Geometry check sheet. Reference: the model listing, model coordinates, mm. Face numbers are marked on the shaded views. A direction names the side the tool comes from. Round coordinates to 2 decimals unless told otherwise and drop trailing zeros. Write each loop counter-clockwise with the first axis right and the second up, starting at its lowest first coordinate (ties: lowest second). Pieces come first, ordered by that corner, then holes.
Item 1: Draft check along X on the marked faces 6, 7 and 8. Enter one of: pulls with the +X half, pulls with the -X half, needs draft (parallel to the pull), parting line crosses it, or undercut.
Item 2: Cross-section at C-C (x = 102.5). Enter the section's corners in (y, z) (3 decimals).
Item 3: Cross-section at B-B (y = 37). Enter the section's corners in (x, z) (3 decimals).
Item 4: Scan lines: probe 1 along Z at (x, y) = (21, 10) (3 decimals); probe 2 along Z at (x, y) = (69, -11) (3 decimals); probe 3 along Y at (x, z) = (11, 49). Record each from-to range of solid material in increasing order.
Item 5: Cross-section at A-A (z = -2.5). Enter the section's corners in (x, y) (3 decimals).
Item 6: Access from +Z, -Z, +X, -X, +Y, -Y to the whole of each face (thin tool, end or side, straight path). Record for the marked faces 1, 2, 3, 4 and 5.
Item 7: Depth check by flat-ended pin: P1, Ø11, axis at y = -7.5, z = 12.5, coming from the +X side (3 decimals); P2, Ø5, axis at y = -15.5, z = 20, coming from the -X side (3 decimals); P3, Ø15.5, axis at x = 20, z = 27, coming from the +Y side; P4, Ø12, axis at x = 36.5, z = 8, coming from the -Y side. Enter the tip coordinate at first touch or a pass-through.
from build123d import *

# Parameters (mm, degrees)
F1_DEPTH = 63.5
F2_DEPTH = 25.4
F0_W     = 25.4
F0_H     = 19.05
F3_DEPTH = 25.4
F4_DEPTH = 7.9375
F6_R     = 6.35


with BuildPart() as f1:
    # F0 (on Front) → F1 (new body, symmetric)
    with BuildSketch(Plane.XZ):
        Polygon((22.225, 9.525), (-41.275, 9.525), (-41.275, -9.525), (41.275, -9.525), (41.275, 9.525), align=None)
    extrude(amount=F1_DEPTH, both=True)

    # F0 (on Front) → F2 (join, symmetric)
    with BuildSketch(Plane.XZ):
        with BuildLine():
            Line((22.225, 27.0002), (22.225, 9.525))
            Line((22.225, 9.525), (41.275, 9.525))
            Line((41.275, 9.525), (41.275, 27.0002))
            ThreePointArc((41.275, 27.0002), (45.9246798487, 38.2255201513), (57.15, 42.8752))
            Line((57.15, 42.8752), (60.325, 42.8752))
            Line((60.325, 42.8752), (60.325, 61.9252))
            Line((60.325, 61.9252), (57.15, 61.9252))
            add(Edge.make_bspline(
                [(56.5114887891, 61.9193627682), (56.7252668459, 61.9225827874), (56.9381101801, 61.9245325067), (57.15, 61.9252)],
                knots=[110.8414409639, 110.8414409639, 110.8414409639, 110.8414409639, 111.5045361635, 111.5045361635, 111.5045361635, 111.5045361635], degree=3))
            ThreePointArc((56.5114887891, 61.9193627682), (32.2295703384, 51.469115188), (22.225, 27.0002))
        make_face()
    extrude(amount=F2_DEPTH, both=True)

    # F0 (on Front) → F3 (join, symmetric)
    with BuildSketch(Plane.XZ):
        with Locations((73.025, 52.4002)):
            Rectangle(F0_W, F0_H)
    extrude(amount=F3_DEPTH, both=True)

    # F0 (on Front) → F4 (join, symmetric)
    with BuildSketch(Plane.XZ):
        with BuildLine():
            add(Edge.make_bspline(
                [(-41.275, 9.525), (-41.0755103707, 25.3485469245), (20.7768493641, 61.3811119099), (56.5114887891, 61.9193627682)],
                knots=[0, 0, 0, 0, 110.8414409639, 110.8414409639, 110.8414409639, 110.8414409639], degree=3))
            Line((-41.275, 9.525), (22.225, 9.525))
            Line((22.225, 9.525), (22.225, 27.0002))
            ThreePointArc((22.225, 27.0002), (32.2295703384, 51.469115188), (56.5114887891, 61.9193627682))
        make_face()
    extrude(amount=F4_DEPTH, both=True)

    # F0 (on Front) → F5 (revolve)
    with BuildSketch(Plane.XZ):
        Polygon((85.725, 66.675), (85.725, 61.9252), (85.725, 42.8752), (85.725, 38.1), (111.125, 38.1), (111.125, 66.675), align=None)
    revolve(axis=Axis((85.725, 0, 52.3875), (0, 0, 1)))

    # F6
    f6_edges = [f1.edges().sort_by_distance(p)[0] for p in [
        (-41.275, -63.5, 0),
        (41.275, -63.5, 0),
        (41.275, 63.5, 0),
        (-41.275, 63.5, 0),
    ]]
    fillet(f6_edges, radius=F6_R)


solid = f1.part
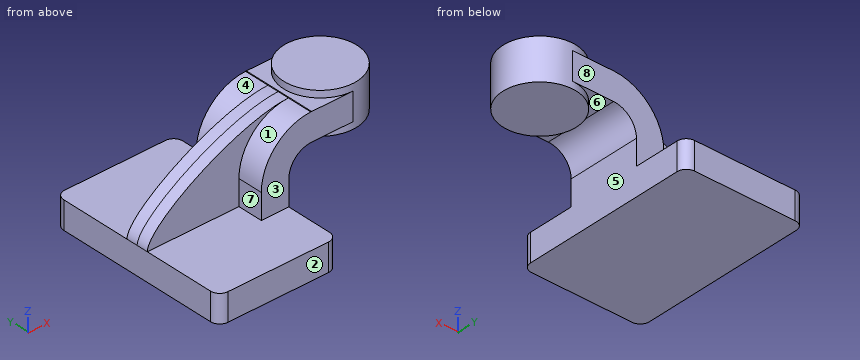
Resolved:
1. face 6: undercut
1. face 7: pulls with the -X half
1. face 8: needs draft
2. outline: (-19.072, 38.1) - (19.072, 38.1) - (19.072, 66.675) - (-19.072, 66.675) - close
3. outline: (-41.275, -9.525) - (41.275, -9.525) - (41.275, 9.525) - (-41.275, 9.525) - close
4. probe 1: z = -9.525 to 9.525
4. probe 2: z = 38.1 to 66.675
4. probe 3: y = -7.94 to 7.94
5. outline: (-41.275, -57.15) arc R6.35 ccw to (-34.925, -63.5) - (34.925, -63.5) arc R6.35 ccw to (41.275, -57.15) - (41.275, 57.15) arc R6.35 ccw to (34.925, 63.5) - (-34.925, 63.5) arc R6.35 ccw to (-41.275, 57.15) - close
6. face 1: +Z, -X, -Y
6. face 2: +Z, -Z, +X, -X, -Y
6. face 3: +Z, +X, -X, -Y
6. face 4: +Z, -X, +Y
6. face 5: -Z, +X, +Y, -Y
7. P1: stops at x = 41.275
7. P2: stops at x = 22.225
7. P3: stops at y = 25.4
7. P4: stops at y = -63.5
